Source: CAD feature listing. Evaluate the final solid. Frame: model axes, mm. A direction names the side the tool comes from. Coordinates: 2 decimals unless noted, no trailing zeros. Write each loop counter-clockwise with the first axis right and the second up, starting at its lowest first coordinate (ties: lowest second). Pieces come first, ordered by that corner, then holes. Notation, with made-up numbers: (-4.5, 22.25) - (37.5, 22.25) arc R15 cw to (37.5, 36.25) - close; hole circle Ø1 at (-8, 12.5). An arc over 180 degrees is marked (long way). One line per question, with ' | ' between items.
from build123d import *
from build123d import SkipClean  # not in build123d's __all__

# Parameters (mm, degrees)
F0_R         = 12.5
F1_DEPTH     = 17
F2_W         = 1.5
F2_H         = 16
F4_R         = 2.5
F5_DEPTH     = 17.001
F6_R         = 9
F6_R_2       = 5
F7_DEPTH     = 8
F8_W         = 4.9303688211
F8_H         = 2
F9_DEPTH     = 0.5
F10_R        = 5
F11_DEPTH    = 8
F12_DEPTH    = 0.5
F13_DEPTH    = 0.5
F14_T4_ANGLE = 359.64


# Not quite as in the source:
# - a fillet or chamfer that OpenCascade refuses, or shapes differently, is made with other operations: its cross-section is extruded or revolved along the edge and cut away or added
# - after a boolean that leaves OpenCascade's solid faulty, fix() repairs it


with BuildPart() as f1:
    # F0 (on Front) → F1 (new body)
    with BuildSketch(Plane.XZ):
        Circle(F0_R)
    extrude(amount=F1_DEPTH)

    # F2 (on Top) → F3 (revolve, cut)
    with BuildSketch(Plane.XY):
        with Locations((-12.75, -8.5)):
            Rectangle(F2_W, F2_H)
    revolve(axis=Axis((0, -8.2131072704, 0), (0, -1, 0)), mode=Mode.SUBTRACT)

    # F4 (on face) → F5 (cut, through all)
    with BuildSketch(Plane(origin=(0, 0, 0), x_dir=(-1, 0, 0), z_dir=(0, 1, 0))):
        Circle(F4_R)
    extrude(amount=-F5_DEPTH, mode=Mode.SUBTRACT)

    # F6 (on face) → F7 (cut)
    with BuildSketch(Plane(origin=(0, 0, 0), x_dir=(-1, 0, 0), z_dir=(0, 1, 0))):
        Circle(F6_R)
        Circle(F6_R_2, mode=Mode.SUBTRACT)
    extrude(amount=-F7_DEPTH, mode=Mode.SUBTRACT)

    # F8 (on face) → F9 (cut)
    with BuildSketch(Plane(origin=(0, 0, 0), x_dir=(-1, 0, 0), z_dir=(0, 1, 0))):
        with Locations((-3.8676508702, 0)):
            Rectangle(F8_W, F8_H)
    extrude(amount=-F9_DEPTH, mode=Mode.SUBTRACT)

    # F10 (on face) → F11 (cut)
    with BuildSketch(Plane.XZ.offset(17)):
        with BuildLine():
            Line((0.75, -8), (0.75, -8.9686955573))
            ThreePointArc((0.75, -8.9686955573), (0, 9), (-0.75, -8.9686955573))
            Line((-0.75, -8.9686955573), (-0.75, -8))
            Line((-0.75, -8), (0.75, -8))
        make_face()
        Circle(F10_R, mode=Mode.SUBTRACT)
    extrude(amount=-F11_DEPTH, mode=Mode.SUBTRACT)

    # F12 (add): a face of the model
    f12_faces = [f1.faces().sort_by_distance(p)[0] for p in [
        (-0.4884023099, 0, 4.8346844466),
    ]]
    with SkipClean():  # cleaning this boolean's faces spoils the solid; the shape is the same uncleaned
        extrude(f12_faces, amount=F12_DEPTH)

    # F13 (add): a face of the model
    f13_faces = [f1.faces().sort_by_distance(p)[0] for p in [
        (-4.8585786438, -17, 0),
    ]]
    extrude(f13_faces, amount=F13_DEPTH)

    add(f1.part.fix(), mode=Mode.REPLACE)

    # F14: chamfer of 1 on 2 edges, made by hand

    # F14_s1 → F14_t2 (revolve, cut)
    with BuildSketch(Plane.XY):
        Polygon((-2.5, -16.5), (-3.5, -17.5), (-2.5, -17.5), align=None)
    revolve(axis=Axis((0, -17.5, 0), (0, 1, 0)), mode=Mode.SUBTRACT)

    # F14_s3 → F14_t4 (revolve, cut)
    with BuildSketch(Plane(origin=(0, 0, 0), x_dir=(0, 1, 0), z_dir=(0.0031415875, 0, 0.9999950652))):
        Polygon((0.5, -3.5), (-0.5, -2.5), (0.5, -2.5), align=None)
    revolve(axis=Axis((0, 0.5, 0), (0, 1, 0)), revolution_arc=F14_T4_ANGLE, mode=Mode.SUBTRACT)


solid = f1.part
Item 1: Cut plane C-C on x = 10.5. Return loops of the section in (y, z).
Check sheet entries:
outline: (-17, -6.78) - (-16.5, -6.78) - (-16.5, -5.81) - (-0.5, -5.81) - (-0.5, -6.78) - (0, -6.78) - (0, 6.78) - (-0.5, 6.78) - (-0.5, 5.81) - (-16.5, 5.81) - (-16.5, 6.78) - (-17, 6.78) - close
Item 2: Pin query (flat end, axial travel): pin 1 Ø4 at (x, z) = (5.5, 5) entering from -Y; pin 2 Ø3 at (y, z) = (-6, -7.5) entering from -X; pin 3 Ø4 at (y, z) = (-8.5, 1.5) entering from +X. Return the tip coordinate at first contact, or that it passes through.
Check sheet entries:
pin 1: y = -17 | pin 2: x = -10.39 | pin 3: x = 12
Item 3: Ray query, line 1 along X through (y, z) = (-6.75, -0.5); line 2 along Z through (x, y) = (0, -3.25); line 3 along Y through (x, z) = (-5, 11.25). Return the intervals inside material, ascending. Write a range as [from, to].
Check sheet entries:
line 1: [-11.99, -8.99], [-4.97, -2.45], [2.45, 4.97], [8.99, 11.99] | line 2: [-12, -9], [-5, -2.5], [2.5, 5], [9, 12] | line 3: [-17, -16.5], [-0.5, 0]
Item 4: Access query for faces 4 (the face through (11.99, -8.39, -0.53)), 5 (the face through (11.923, -16.746, 3.755)), 6 (the face through (-0.75, -13.1, -8.5)), 7 (the face through (-4, -8, -4)). Directions: +Z, -Z, +X, -X, +Y, -Y. A direction counts if a zero-diameter tool reaches every point of the face in a straight line with its end or side. Return the directions, or none.
Check sheet entries:
face 4: none | face 5: +Y, -Y | face 6: -Y | face 7: +Y
Item 5: Cut plane A-A on y = -11. Return loops of the section in (x, z).
Check sheet entries:
outline: circle Ø24 at (0, 0); circle Ø10 at (0, 0); hole circle Ø5 at (0, 0); hole (-0.75, -8.97) - (-0.75, -8) - (0.75, -8) - (0.75, -8.97) arc R9 ccw (long way) to start
Item 6: Cut plane B-B on z = -6.5. Return loops of the section in (x, y).
Check sheet entries:
outline: (-10.68, -17) - (-6.22, -17) - (-6.22, -9) - (6.22, -9) - (6.22, -17) - (10.68, -17) - (10.68, -16.5) - (10.09, -16.5) - (10.09, -0.5) - (10.68, -0.5) - (10.68, 0) - (6.22, 0) - (6.22, -8) - (-6.22, -8) - (-6.22, 0) - (-10.68, 0) - (-10.68, -0.5) - (-10.09, -0.5) - (-10.09, -16.5) - (-10.68, -16.5) - close
Item 7: Cut plane D-D on z = 4.5. Return loops of the section in (x, y), and give its area (3 significant figures).
Check sheet entries:
outline: (-11.66, -17) - (-7.79, -17) - (-7.79, -9) - (-2.18, -9) - (-2.18, -17.5) - (2.18, -17.5) - (2.18, -9) - (7.79, -9) - (7.79, -17) - (11.66, -17) - (11.66, -16.5) - (11.12, -16.5) - (11.12, -0.5) - (11.66, -0.5) - (11.66, 0) - (7.79, 0) - (7.79, -8) - (2.18, -8) - (2.18, 0.5) - (-2.18, 0.5) - (-2.18, -8) - (-7.79, -8) - (-7.79, 0) - (-11.66, 0) - (-11.66, -0.5) - (-11.12, -0.5) - (-11.12, -16.5) - (-11.66, -16.5) - close | area: 204 mm²
Item 8: Mould query, pull axis Y, two halves, no side actions, for faces 1 (the face through (7, -0.5, -10)), 2 (the face through (1.172, -3.944, 8.923)), 3 (the face through (2.2, -17.5, -3.3)). Classes: pulls with the +Y half, pulls with the -Y half, needs draft (parallel to the pull), parting line crosses it, or undercut.
Check sheet entries:
face 1: undercut | face 2: needs draft | face 3: pulls with the -Y half
